Could you check a few things on this model? Use its own coordinates, in mm. A direction names the side the tool comes from. Round coordinates to 2 decimals unless told otherwise and drop trailing zeros. Order: outer loops, then holes, each group sorted by start corner. A loop starts at its lowest first (then second) coordinate and runs counter-clockwise, first axis right, second up. Notation, with made-up numbers: (28, 44.5) - (44, 44.5) arc R25 cw to (44, 58.5) - close; hole circle Ø4 at (83.5, 81). An arc over 180 degrees is marked (long way). Return JSON: item names as keys, results as strings. Group by question number.
from build123d import *

# Parameters (mm, degrees)
SKETCH1_R           = 75
BOSS_EXTRUDE1_DEPTH = 10
SKETCH2_R           = 5
CUT_EXTRUDE1_DEPTH  = 10
SKETCH3_R           = 20
CUT_EXTRUDE2_DEPTH  = 10
BOSS_EXTRUDE2_START = 150
SKETCH4_R           = 25
SKETCH4_R_2         = 20
BOSS_EXTRUDE2_DEPTH = 150


with BuildPart() as part:
    # Sketch1 → Boss-Extrude1 (new body)
    with BuildSketch(Plane(origin=(0, 0, 0), x_dir=(1, 0, 0), z_dir=(0, 1, 0))):
        with Locations(Location((0, 0, 0), (0, 0, 270))):
            Circle(SKETCH1_R)
    extrude(amount=BOSS_EXTRUDE1_DEPTH)

    # Sketch2 → Cut-Extrude1 (cut)
    with BuildSketch(Plane(origin=(0, 10, 0), x_dir=(1, 0, 0), z_dir=(0, 1, 0))):
        with Locations(Location((0, 57.614814887, 0), (0, 0, 270))):
            Circle(SKETCH2_R)
        with Locations(Location((54.794945134, 17.803956928, 0), (0, 0, 270))):
            Circle(SKETCH2_R)
        with Locations(Location((33.865138504, -46.611364372, 0), (0, 0, 270))):
            Circle(SKETCH2_R)
        with Locations(Location((-33.865138504, -46.611364372, 0), (0, 0, 270))):
            Circle(SKETCH2_R)
        with Locations(Location((-54.794945134, 17.803956928, 0), (0, 0, 270))):
            Circle(SKETCH2_R)
    extrude(amount=-CUT_EXTRUDE1_DEPTH, mode=Mode.SUBTRACT)

    # Sketch3 → Cut-Extrude2 (cut)
    with BuildSketch(Plane(origin=(0, 10, 0), x_dir=(1, 0, 0), z_dir=(0, 1, 0))):
        with Locations(Location((0, 0, 0), (0, 0, 270))):
            Circle(SKETCH3_R)
    extrude(amount=-CUT_EXTRUDE2_DEPTH, mode=Mode.SUBTRACT)

    # Sketch4 → Boss-Extrude2 (add)
    with BuildSketch(Plane(origin=(0, 10, 0), x_dir=(1, 0, 0), z_dir=(0, 1, 0)).offset(BOSS_EXTRUDE2_START)):
        with Locations(Location((0, 0, 0), (0, 0, 270))):
            Circle(SKETCH4_R)
        with Locations(Location((0, 0, 0), (0, 0, 270))):
            Circle(SKETCH4_R_2, mode=Mode.SUBTRACT)
    extrude(amount=-BOSS_EXTRUDE2_DEPTH)


solid = part.part
1) Will these pins go through, and if not, where does the flat tip stop? pin 1 (5 mm diameter, centred on y = 115, z = -11.5, fed in from -X); pin 2 (9 mm diameter, centred on x = 54.79, z = -17.8, fed in from -Y); pin 3 (2 mm diameter, centred on x = 51.5, z = -53.5, fed in from +Y); pin 4 (5 mm diameter, centred on x = -31, z = -33, fed in from -Y).
2) I want a section at B-B, the plane x = 0. List the corners of the cut face in (y, z) for me.
3) I want a section at A-A, the plane z = 0. List the corners of the cut face in (x, y) for me, plus the area to 3 significant figures.
4) I want a section at C-C, the plane y = 146. List the corners of the cut face in (x, z) for me, plus the area to 3 significant figures.
5) For faces 1 (the flat face through (17, 160, -11)), 2 (the cylindrical face through (7.509, 86.05, 23.846)), which set-ups out of +Z, -Z, +X, -X, +Y, -Y let a thin tool reach every point of the face, with its end or its side?
6) I want a section at D-D, the plane z = 15. List the corners of the cut face in (x, y) for me, plus the area to 3 significant figures.
7) We'd pull the mould along Z, two halves only. Please class faces 3 (the flat face through (18, 10, -18)), 4 (the cylindrical face through (-53.293, 5.07, -13.035)), 5 (the cylindrical face through (-45.636, 4.93, -59.517)): +Z half, -Z half, draft (parallel to the pull), parting line (faces both ways), or undercut.
8) If I drill on line 1 along X through (y, z) = (106, 0); line 2 along Y through (x, z) = (50, 7.5); line 3 along Z through (x, y) = (56, 9.5), over which ranges is the centre line in solid material (lowest first)? Write a range as from..to.
Outcome:
{
 "1": {"pin 1": "x = -23.32", "pin 2": "through", "pin 3": "y = 10", "pin 4": "y = 0"},
 "2": {"outline": "(0, -75) - (10, -75) - (10, -62.61) - (0, -62.61) - close; (0, -52.61) - (10, -52.61) - (10, -25) - (160, -25) - (160, -20) - (0, -20) - close; (0, 20) - (160, 20) - (160, 25) - (10, 25) - (10, 75) - (0, 75) - close"},
 "3": {"outline": "(-75, 0) - (-20, 0) - (-20, 160) - (-25, 160) - (-25, 10) - (-75, 10) - close; (20, 0) - (75, 0) - (75, 10) - (25, 10) - (25, 160) - (20, 160) - close", "area": "2,600 mm^2"},
 "4": {"outline": "circle Ø50 at (0, 0); hole circle Ø40 at (0, 0)", "area": "707 mm^2"},
 "5": {"face 1": "+Z, -Z, +X, -X, +Y", "face 2": "+Y"},
 "6": {"outline": "(-73.48, 0) - (-13.23, 0) - (-13.23, 160) - (-20, 160) - (-20, 10) - (-73.48, 10) - close; (13.23, 0) - (73.48, 0) - (73.48, 10) - (20, 10) - (20, 160) - (13.23, 160) - close", "area": "3,240 mm^2"},
 "7": {"face 3": "draft", "face 4": "undercut", "face 5": "parting line"},
 "8": {"line 1": "-25..-20, 20..25", "line 2": "0..10", "line 3": "-49.89..-22.66, -12.95..49.89"}
}
